CAD build for the part. Positions are in the model's coordinates, mm. A direction names the side the tool comes from. Give positions to 0.01 mm unless a question says otherwise; leave off trailing zeros. Write each loop counter-clockwise with the first axis right and the second up, starting at its lowest first coordinate (ties: lowest second). Pieces come first, ordered by that corner, then holes. Notation, with made-up numbers: (-19.75, 32.25) - (16.25, 32.25) arc R23 cw to (16.25, 54.25) - close; hole circle Ø3 at (-3, 75). An arc over 180 degrees is marked (long way). Answer as a JSON object with one key per item and string values.
from build123d import *

# Parameters (mm, degrees)
SKETCH_1_W      = 32
SKETCH_1_H      = 23
EXTRUDE_1_DEPTH = 0.5
EXTRUDE_3_DEPTH = 5
EXTRUDE_4_DEPTH = 6.6


with BuildPart() as part:
    # 草图1 → 凸台-拉伸1 (new body)
    with BuildSketch(Plane(origin=(0, 0, 0), x_dir=(1, 0, 0), z_dir=(0, 1, 0))):
        Rectangle(SKETCH_1_W, SKETCH_1_H)
    extrude(amount=EXTRUDE_1_DEPTH)

    # 草图5 → 凸台-拉伸3 (add)
    with BuildSketch(Plane.ZY.offset(9)):
        with BuildLine():
            Line((-11.5, 0), (-11.5, 14))
            ThreePointArc((-11.5, 14), (-18.5, 7), (-11.5, 0))
        make_face()
    extrude(amount=-EXTRUDE_3_DEPTH)

    # 草图7 → 凸台-拉伸4 (add)
    with BuildSketch(Plane.ZY.offset(14)):
        with BuildLine():
            Line((11.473319553, 0), (11.5, 13.999974577))
            ThreePointArc((11.5, 13.999974577), (18.486647065, 6.986647065), (11.473319553, 0))
        make_face()
    extrude(amount=-EXTRUDE_4_DEPTH)


solid = part.part
(1) Pull direction Z, two halves, no side cores. Call faces 1 (the face through (-6.54, 7.15, -18.5)), 2 (the face through (-7.4, 7, 14)), 3 (the face through (-7, 7, -11.5)): pulls with the +Z half, pulls with the -Z half, needs draft (parallel to the pull), parting line crosses it, or undercut.
Answer key:
{"face 1": "pulls with the -Z half", "face 2": "needs draft", "face 3": "undercut"}
(2) Flat gauge pins, fed straight in: P1, Ø7.5, axis at y = 5.5, z = 16, coming from the +X side; P2, Ø1.5, axis at y = 2, z = 7, coming from the +X side; P3, Ø0.6, axis at x = 1, y = 0.5, coming from the +Z side; P4, Ø18.5, axis at x = 6, z = -1, coming from the +Y side. Where does each tip first touch, or does it go through?
Answer key:
{"P1": "stops at x = -7.4", "P2": "passes through", "P3": "stops at z = 11.5", "P4": "stops at y = 0.5"}
(3) Saw through at C-C, the plane z = 0.5. Give the cut face in (x, y), and give its area (3 significant figures).
Answer key:
{"outline": "(-16, 0) - (16, 0) - (16, 0.5) - (-16, 0.5) - close", "area": "16.0 mm²"}
(4) Saw through at D-D, the plane y = 6.25. Give the cut face in (x, z).
Answer key:
{"outline": "(-14, 11.49) - (-7.4, 11.49) - (-7.4, 18.45) - (-14, 18.45) - close; (-9, -18.46) - (-4, -18.46) - (-4, -11.5) - (-9, -11.5) - close"}
(5) Saw through at B-B, the plane x = -5.5. Give the cut face in (y, z), and give its area (3 significant figures).
Answer key:
{"outline": "(0, -11.5) arc R7 ccw to (14, -11.5) - (0.5, -11.5) - (0.5, 11.5) - (0, 11.5) - close", "area": "88.5 mm²"}
(6) Saw through at A-A, the plane y = 1.5. Give the cut face in (x, z), and give its area (3 significant figures).
Answer key:
{"outline": "(-14, 11.48) - (-7.4, 11.48) - (-7.4, 15.82) - (-14, 15.82) - close; (-9, -15.83) - (-4, -15.83) - (-4, -11.5) - (-9, -11.5) - close", "area": "50.3 mm²"}
(7) Probe L1, parallel to Y at x = -12, z = -7; L2, parallel to X at y = 2.25, z = -15.5; L3, parallel to X at y = 13.25, z = 12. List the from-to ranges inside material, lowest first. Write a range as [from, to].
Answer key:
{"L1": "y = [0, 0.5]", "L2": "x = [-9, -4]", "L3": "x = [-14, -7.4]"}
(8) 3-axis set-ups, long thin cutter, end or side, ignore diameter. For faces 4 (the face through (0, 0, 0)), 5 (the face through (-9, 7, -14)): which of +Z, -Z, +X, -X, +Y, -Y reach the whole face in a straight line?
Answer key:
{"face 4": "+Z, -Z, +X, -X, -Y", "face 5": "-Z, -X, +Y, -Y"}
